```python
from build123d import *

# Parameters (mm, degrees)
SKETCH1_W           = 100
SKETCH1_H           = 100
BOSS_EXTRUDE1_DEPTH = 4
SKETCH2_R           = 1.75
CUT_EXTRUDE1_DEPTH  = 10
SKETCH3_OUTSIDE_W   = 130.296
SKETCH3_OUTSIDE_H   = 130.296
SKETCH3_OUTSIDE_R   = 50
CUT_EXTRUDE2_DEPTH  = 10
SKETCH4_R           = 2.5
CUT_EXTRUDE3_DEPTH  = 10
SKETCH5_R           = 4.75
CUT_EXTRUDE4_DEPTH  = 2
CHAMFER1_SIZE       = 2


with BuildPart() as part:
    # Sketch1 → Boss-Extrude1 (new body)
    with BuildSketch(Plane(origin=(0, 0, 0), x_dir=(1, 0, 0), z_dir=(0, 1, 0))):
        Rectangle(SKETCH1_W, SKETCH1_H)
    extrude(amount=BOSS_EXTRUDE1_DEPTH)

    # Sketch2 → Cut-Extrude1 (cut)
    with BuildSketch(Plane(origin=(0, 4, 0), x_dir=(1, 0, 0), z_dir=(0, 1, 0))):
        with Locations(Location((-34, 0, 0), (0, 0, 270))):
            Circle(SKETCH2_R)
        with Locations(Location((-24.04163056, 24.04163056, 0), (0, 0, 270))):
            Circle(SKETCH2_R)
        with Locations(Location((0, 34, 0), (0, 0, 270))):
            Circle(SKETCH2_R)
        with Locations(Location((24.04163056, 24.04163056, 0), (0, 0, 270))):
            Circle(SKETCH2_R)
        with Locations(Location((34, 0, 0), (0, 0, 270))):
            Circle(SKETCH2_R)
        with Locations(Location((24.04163056, -24.04163056, 0), (0, 0, 270))):
            Circle(SKETCH2_R)
        with Locations(Location((0, -34, 0), (0, 0, 270))):
            Circle(SKETCH2_R)
        with Locations(Location((-24.04163056, -24.04163056, 0), (0, 0, 270))):
            Circle(SKETCH2_R)
    extrude(amount=-CUT_EXTRUDE1_DEPTH, mode=Mode.SUBTRACT)

    # Sketch3 outside → Cut-Extrude2 (cut)
    with BuildSketch(Plane(origin=(0, 4, 0), x_dir=(1, 0, 0), z_dir=(0, 1, 0))):
        Rectangle(SKETCH3_OUTSIDE_W, SKETCH3_OUTSIDE_H)
        with Locations(Location((0, 0, 0), (0, 0, 270))):
            Circle(SKETCH3_OUTSIDE_R, mode=Mode.SUBTRACT)
    extrude(amount=-CUT_EXTRUDE2_DEPTH, mode=Mode.SUBTRACT)

    # Sketch4 → Cut-Extrude3 (cut)
    with BuildSketch(Plane(origin=(0, 4, 0), x_dir=(1, 0, 0), z_dir=(0, 1, 0))):
        with BuildLine():
            ThreePointArc((-18.177463037, 43.884277794), (-19.530453288, 40.617870382), (-16.264045876, 39.264880132))
            Line((-16.264045876, 39.264880132), (-18.177463037, 43.884277794))
        make_face()
        with BuildLine():
            Line((-18.177463037, 43.884277794), (-16.264045876, 39.264880132))
            ThreePointArc((-16.264045876, 39.264880132), (-15.142080426, 40.18565338), (-14.720754456, 41.574578963))
            ThreePointArc((-14.720754456, 41.574578963), (-15.831828874, 43.653252994), (-18.177463037, 43.884277794))
        make_face()
        with Locations(Location((41.574578963, 17.220754456, 0), (0, 0, 270))):
            Circle(SKETCH4_R)
        with Locations(Location((-41.574578963, -17.220754456, 0), (0, 0, 270))):
            Circle(SKETCH4_R)
        with Locations(Location((17.220754456, -41.574578963, 0), (0, 0, 270))):
            Circle(SKETCH4_R)
    extrude(amount=-CUT_EXTRUDE3_DEPTH, mode=Mode.SUBTRACT)

    # Sketch5 → Cut-Extrude4 (cut)
    with BuildSketch(Plane(origin=(0, 4, 0), x_dir=(1, 0, 0), z_dir=(0, 1, 0))):
        with Locations(Location((0, -34, 0), (0, 0, 270))):
            Circle(SKETCH5_R)
        with Locations(Location((24.04163056, -24.04163056, 0), (0, 0, 270))):
            Circle(SKETCH5_R)
        with Locations(Location((34, 0, 0), (0, 0, 270))):
            Circle(SKETCH5_R)
        with Locations(Location((24.04163056, 24.04163056, 0), (0, 0, 270))):
            Circle(SKETCH5_R)
        with Locations(Location((-24.04163056, -24.04163056, 0), (0, 0, 270))):
            Circle(SKETCH5_R)
        with Locations(Location((-34, 0, 0), (0, 0, 270))):
            Circle(SKETCH5_R)
        with Locations(Location((-24.04163056, 24.04163056, 0), (0, 0, 270))):
            Circle(SKETCH5_R)
        with Locations(Location((0, 34, 0), (0, 0, 270))):
            Circle(SKETCH5_R)
    extrude(amount=-CUT_EXTRUDE4_DEPTH, mode=Mode.SUBTRACT)

    # Chamfer1
    chamfer1_edges = [part.edges().sort_by_distance(p)[0] for p in [
        (0, 2, 32.25),
        (0, 2, -35.75),
        (-24.04163056, 2, -25.79163056),
        (-34, 2, -1.75),
        (24.04163056, 2, 22.29163056),
        (34, 2, -1.75),
        (24.04163056, 2, -25.79163056),
        (-24.04163056, 2, 22.29163056),
    ]]
    chamfer(chamfer1_edges, length=CHAMFER1_SIZE - 0.0001)  # a hair under: the kernel refuses the full size


solid = part.part
```
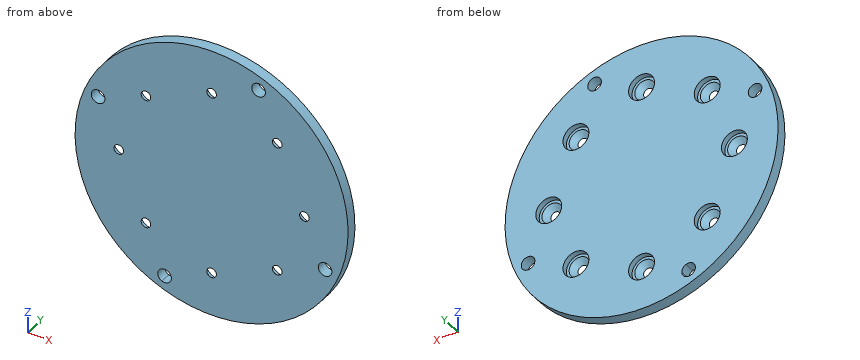
Geometry: final body of the model. Coordinates: model frame, mm. Coordinates: 2 decimals unless noted, no trailing zeros.
Item 1: Contact query for flat-ended pins moving along their axis: P1, Ø5.5, axis at x = -24.04, z = -24.04, coming from the +Y side; P2, Ø1.5, axis at y = 0.5, z = 13.5, coming from the +X side; P3, Ø1.5, axis at x = -14, y = 2, coming from the +Z side. Output: stop coordinate, or through.
Answer:
P1: stops at y = 1
P2: stops at x = 48.35
P3: stops at z = 48.21
Item 2: Material intervals for line 1 along Z through (x, y) = (22, 3.6); line 2 along X through (y, z) = (0.7, -24); line 3 along X through (y, z) = (2.55, 42.5), sorted ascending.
Answer:
line 1: z = -44.9 to -28.33, -19.75 to 19.75, 28.33 to 44.9
line 2: x = -43.86 to -26.49, -21.59 to 21.59, 26.49 to 43.86
line 3: x = -26.34 to 14.9, 19.54 to 26.34
Item 3: Section query A-A (z = 0). State how many separate pieces and enclosed holes the cut face has, then the cut area to 3 significant figures.
Answer:
separate pieces: 3
enclosed holes: 0
area: 340 mm2
